The model under review builds one solid part; all positions refer to its coordinate system, in mm. Face numbers are marked on the shaded views. A direction names the side the tool comes from. Coordinates: 2 decimals unless noted, no trailing zeros. Write each loop counter-clockwise with the first axis right and the second up, starting at its lowest first coordinate (ties: lowest second). Pieces come first, ordered by that corner, then holes. Notation, with made-up numbers: (-29, 19.25) - (2, 19.25) arc R21 cw to (2, 28.25) - close; hole circle Ø4 at (-6, 77.5). An arc over 180 degrees is marked (long way). Use one line per item in the form item = value. Start each with the question number.
```python
from build123d import *

# Parameters (mm, degrees)
SKETCH031_W     = 10.922
SKETCH031_H     = 19.05
PAD002_DEPTH    = 5.461
SKETCH033_R     = 3.0099
POCKET003_DEPTH = 7.239
SKETCH035_R     = 1.651
POCKET004_DEPTH = 19.051
SKETCH036_R     = 2.7305
POCKET005_DEPTH = 7.62
SKETCH039_R     = 0.889
POCKET006_DEPTH = 19.082657
CHAMFER_SIZE    = 1.016


with BuildPart() as part:
    # Sketch031 → Pad002 (new body, symmetric)
    with BuildSketch(Plane.YZ):
        with Locations((-9.779, 28.194)):
            Rectangle(SKETCH031_W, SKETCH031_H)
    extrude(amount=PAD002_DEPTH, both=True)

    # Sketch033 (on Face1 of Pad002) → Pocket003 (cut)
    with BuildSketch(Plane(origin=(0, 0, 37.719), x_dir=(0, -1, 0), z_dir=(0, 0, 1))):
        with Locations((9.779, 0)):
            Circle(SKETCH033_R)
    extrude(amount=-POCKET003_DEPTH, mode=Mode.SUBTRACT)

    # Sketch035 (on Face1 of Pad002) → Pocket004 (cut, through all)
    with BuildSketch(Plane(origin=(0, 0, 37.719), x_dir=(0, -1, 0), z_dir=(0, 0, 1))):
        with Locations((9.779, 0)):
            Circle(SKETCH035_R)
    extrude(amount=-POCKET004_DEPTH, mode=Mode.SUBTRACT)

    # Sketch036 (on Face7 of Pocket004) → Pocket005 (cut)
    with BuildSketch(Plane.YX.offset(-18.669)):
        with Locations((-9.779, 0)):
            Circle(SKETCH036_R)
    extrude(amount=-POCKET005_DEPTH, mode=Mode.SUBTRACT)

    # Sketch039 → Pocket006 (cut, through all)
    with BuildSketch(Plane(origin=(0, 0, 18.669), x_dir=(0.003059, 0.999994, 0.001528), z_dir=(-0.001528, 0.001533, -0.999998))):
        with Locations((-11.853333, 5.461)):
            Circle(SKETCH039_R)
        with Locations((-7.704667, 5.461)):
            Circle(SKETCH039_R)
    extrude(amount=-POCKET006_DEPTH, mode=Mode.SUBTRACT)

    # Chamfer
    chamfer_edges = [part.edges().sort_by_distance(p)[0] for p in [
        (-5.461, -4.318, 28.194),
        (-5.461, -15.24, 28.194),
        (5.461, -15.24, 28.194),
        (5.461, -4.318, 28.194),
    ]]
    chamfer(chamfer_edges, length=CHAMFER_SIZE)


with BuildPart() as part_1:
    # Body001 placement: moved
    add(part.part.moved(Location((0, -3, 0))))


solid = part_1.part
```
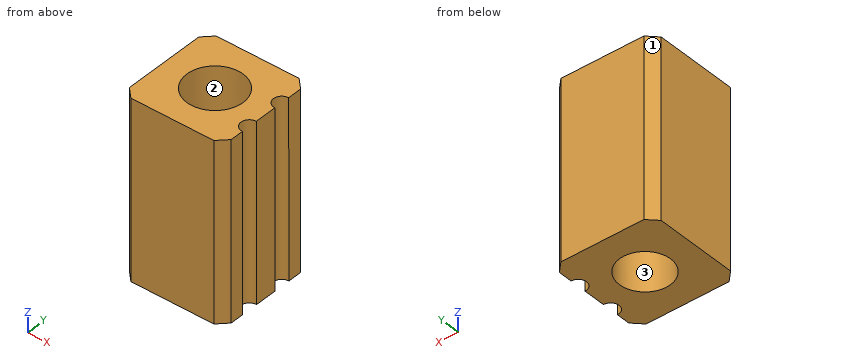
1. For the marked faces 1, 2 and 3, list the 3-axis set-ups (+Z, -Z, +X, -X, +Y, -Y) from which the entire face can be reached by the end or side of a thin tool; tool diameter is ignored.
2. For P1, Ø3, axis at x = -0.5, y = -11.5, coming from the +Z side; P2, Ø1.6, axis at x = -1, y = -13.5, coming from the -Z side, all flat-tipped, find the tip position at first contact; note any pin that passes through.
3. For L1, parallel to X at y = -12.75, z = 34.25; L2, parallel to X at y = -12.75, z = 29; L3, parallel to Z at x = -1.5, y = -14, list the stretches that pass through material, from the lowest coordinate up.
4. Take a section at A-A (x = 0). State the section outline as (y, z) points.
5. Take a section at B-B (y = -13). State the section outline as (x, z) points, plus the area to 3 significant figures.
Returned:
q1.face_1 = +Z, -Z, -X, +Y
q1.face_2 = +Z
q1.face_3 = -Z
q2.P1 = 30.48
q2.P2 = 26.29
q3.L1 = -5.46 to -3.01, 3.01 to 5.46
q3.L2 = -5.46 to -1.65, 1.65 to 5.46
q3.L3 = 26.29 to 30.48
q4.outline = (-18.24, 18.67) - (-15.51, 18.67) - (-15.51, 26.29) - (-14.43, 26.29) - (-14.43, 30.48) - (-15.79, 30.48) - (-15.79, 37.72) - (-18.24, 37.72) - close; (-11.13, 26.29) - (-10.05, 26.29) - (-10.05, 18.67) - (-7.32, 18.67) - (-7.32, 37.72) - (-9.77, 37.72) - (-9.77, 30.48) - (-11.13, 30.48) - close
q5.outline = (-5.46, 18.67) - (-2.72, 18.67) - (-2.72, 26.29) - (-1.64, 26.29) - (-1.64, 30.48) - (-3, 30.48) - (-3, 37.72) - (-5.46, 37.72) - close; (1.64, 26.29) - (2.72, 26.29) - (2.72, 18.67) - (5.46, 18.67) - (5.46, 37.72) - (3, 37.72) - (3, 30.48) - (1.64, 30.48) - close
q5.area = 109 mm²
